Geometry check sheet. Reference: the model listing, model coordinates, mm. Face numbers are marked on the shaded views. Coordinates: 2 decimals unless noted, no trailing zeros. Write each loop counter-clockwise with the first axis right and the second up, starting at its lowest first coordinate (ties: lowest second). Pieces come first, ordered by that corner, then holes. Notation, with made-up numbers: (-39, -29.75) -> (-17, -29.75) arc R14 cw to (-17, -25.75) -> close; hole circle Ø7 at (28, -18.75). An arc over 180 degrees is marked (long way). Answer in a Markdown table with one row per item. Add a question column.
1. Depth check by flat-ended pin: P1, Ø8, axis at y = -8.5, z = 5.5, coming from the -X side; P2, Ø4, axis at y = -10, z = 8, coming from the +X side. Enter the tip coordinate at first touch or a pass-through.
2. Cross-section at A-A on z = -2. Record the cut outline in (x, y).
3. Mould release check, pull along Z, two halves, no side actions. Record for the marked faces 1, 2 and 3: pulls with the +Z half, pulls with the -Z half, needs draft (parallel to the pull), parting line crosses it, or undercut.
4. Scan lines: L1, parallel to X at y = -6.5, z = 4; L2, parallel to X at y = -5.75, z = 1; L3, parallel to Z at x = -26.5, y = -3.5. Record each from-to range of solid material in increasing order. Write a range as from..to.
5. Cross-section at C-C on y = -11.75. Record the cut outline in (x, z).
6. Cross-section at D-D on z = 3.25. Record the cut outline in (x, y).
7. Cross-section at B-B on x = 20.5. Record the cut outline in (y, z), and give its area (3 significant figures).
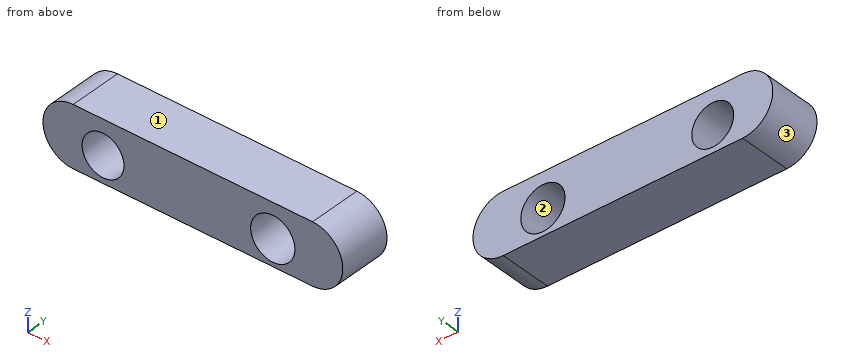
```python
from build123d import *

# Parameters (mm, degrees)
F0_R     = 5.977337
F0_R_2   = 6.310388
F1_DEPTH = 15


with BuildPart() as f1:
    # F0 (on Front) → F1 (new body)
    with BuildSketch(Plane.XZ):
        Polygon((33.567898, 9.772932), (0, 9.772932), (-34.70099, 9.772932), (-34.70099, -7.506745), (33.567898, -7.506745), align=None)
        with Locations((-26.202789, 0)):
            Circle(F0_R, mode=Mode.SUBTRACT)
        with Locations((22.23696, 0)):
            Circle(F0_R_2, mode=Mode.SUBTRACT)
        with BuildLine():
            Line((-34.70099, -7.506745), (-34.70099, 9.772932))
            ThreePointArc((-34.70099, 9.772932), (-43.340828, 1.133094), (-34.70099, -7.506745))
        make_face()
        with BuildLine():
            ThreePointArc((33.567898, -7.506745), (42.207737, 1.133094), (33.567898, 9.772932))
            Line((33.567898, 9.772932), (33.567898, -7.506745))
        make_face()
    extrude(amount=F1_DEPTH)


solid = f1.part
```
Results found:
| question | item | result |
|---|---|---|
| 1 | P1 | stops at x = -43.33 |
| 1 | P2 | stops at x = 40.71 |
| 2 | outline | (-42.75, -15) -> (-31.84, -15) -> (-31.84, 0) -> (-42.75, 0) -> close; (-20.57, -15) -> (16.25, -15) -> (16.25, 0) -> (-20.57, 0) -> close; (28.22, -15) -> (41.62, -15) -> (41.62, 0) -> (28.22, 0) -> close |
| 3 | face 1 | pulls with the +Z half |
| 3 | face 2 | undercut |
| 3 | face 3 | parting line crosses it |
| 4 | L1 | x = -42.85..-30.64, -21.76..17.36, 27.12..41.72 |
| 4 | L2 | x = -43.34..-32.1, -20.31..16.01, 28.47..42.21 |
| 4 | L3 | z = -7.51..-5.97, 5.97..9.77 |
| 5 | outline | (-34.7, -7.51) -> (33.57, -7.51) arc R8.64 ccw to (33.57, 9.77) -> (-34.7, 9.77) arc R8.64 ccw to start; hole circle Ø11.95 at (-26.2, 0); hole circle Ø12.62 at (22.24, 0) |
| 6 | outline | (-43.08, -15) -> (-31.22, -15) -> (-31.22, 0) -> (-43.08, 0) -> close; (-21.19, -15) -> (16.83, -15) -> (16.83, 0) -> (-21.19, 0) -> close; (27.65, -15) -> (41.94, -15) -> (41.94, 0) -> (27.65, 0) -> close |
| 7 | outline | (-15, -7.51) -> (0, -7.51) -> (0, -6.07) -> (-15, -6.07) -> close; (-15, 6.07) -> (0, 6.07) -> (0, 9.77) -> (-15, 9.77) -> close |
| 7 | area | 77.2 mm^2 |
